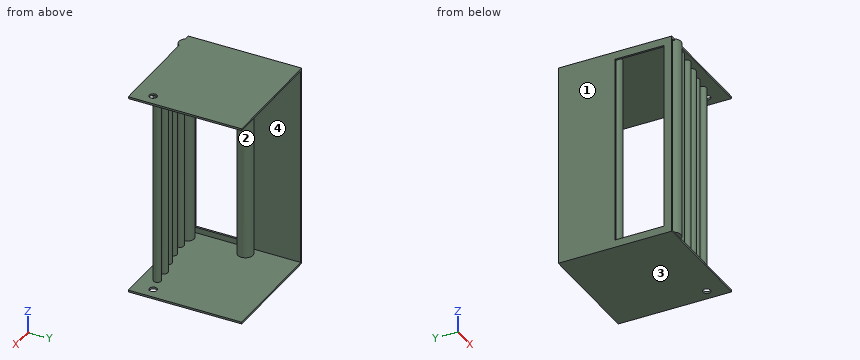
```python
from build123d import *

# Parameters (mm, degrees)
SKETCH1_W               = 381
SKETCH1_H               = 685.8
BOSS_EXTRUDE1_DEPTH     = 381
SHELL1_T                = -6.35
SKETCH4_R               = 12.7
CUT_EXTRUDE1_DEPTH      = 1
CUT_EXTRUDE1_DEPTH_BACK = 686.8
SKETCH5_R               = 12.7
BOSS_EXTRUDE3_DEPTH     = 679.45
SKETCH6_R               = 25.4
BOSS_EXTRUDE4_DEPTH     = 679.45
CUT_EXTRUDE3_REACH      = 8.35
SKETCH7_W               = 635
SKETCH7_H               = 165.1


with BuildPart() as part:
    # Sketch1 → Boss-Extrude1 (new body)
    with BuildSketch(Plane(origin=(0, 0, 0), x_dir=(1, 0, 0), z_dir=(0, 1, 0))):
        with Locations((190.5, 342.9)):
            Rectangle(SKETCH1_W, SKETCH1_H)
    extrude(amount=BOSS_EXTRUDE1_DEPTH)

    # Shell1
    shell1_openings = [part.faces().sort_by_distance(p)[0] for p in [
        (190.5, 381, -342.9),
        (190.5, 0, -342.9),
        (381, 190.5, -342.9),
    ]]
    offset(amount=SHELL1_T, openings=shell1_openings, kind=Kind.INTERSECTION)

    # Sketch4 → Cut-Extrude1 (cut, two sides)
    with BuildSketch(Plane.XY) as cut_extrude1_sk:
        with Locations((342.9, 63.5)):
            Circle(SKETCH4_R)
    extrude(amount=CUT_EXTRUDE1_DEPTH, mode=Mode.SUBTRACT)
    extrude(cut_extrude1_sk.sketch, amount=-CUT_EXTRUDE1_DEPTH_BACK, mode=Mode.SUBTRACT)

    # Sketch5 → Boss-Extrude3 (add)
    with BuildSketch(Plane.XY):
        with Locations((292.1, 50.8)):
            Circle(SKETCH5_R)
        with Locations((190.5, 32.743756917)):
            Circle(SKETCH5_R)
        with Locations((88.9, 19.34192219)):
            Circle(SKETCH5_R)
        with Locations((241.3, 46.355575893)):
            Circle(SKETCH5_R)
        with Locations((139.7, 23.786346297)):
            Circle(SKETCH5_R)
    extrude(amount=-BOSS_EXTRUDE3_DEPTH)

    # Sketch6 → Boss-Extrude4 (add)
    with BuildSketch(Plane.XY):
        with Locations((38.1, 14.897498083)):
            Circle(SKETCH6_R)
        with Locations((38.1, 211.747498083)):
            Circle(SKETCH6_R)
    extrude(amount=-BOSS_EXTRUDE4_DEPTH)

    # Sketch7 → Cut-Extrude3 (cut, up to next)
    with BuildSketch(Plane(origin=(6.35, 0, 0), x_dir=(0, 0, -1), z_dir=(1, 0, 0)), mode=Mode.PRIVATE) as cut_extrude3_sk1:
        with Locations((342.9, 107.95)):
            Rectangle(SKETCH7_W, SKETCH7_H)
    cut_extrude3_tool1 = extrude(cut_extrude3_sk1.sketch, amount=-CUT_EXTRUDE3_REACH, mode=Mode.PRIVATE) & part.part
    add(cut_extrude3_tool1.solids().sort_by_distance((6.35, 107.95, -342.9))[0], mode=Mode.SUBTRACT)


solid = part.part
```
Source: CAD feature listing. Evaluate the final solid. Frame: model axes, mm. Face numbers are marked on the shaded views. A direction names the side the tool comes from. Give positions to 0.01 mm unless a question says otherwise; leave off trailing zeros. Write each loop counter-clockwise with the first axis right and the second up, starting at its lowest first coordinate (ties: lowest second). Pieces come first, ordered by that corner, then holes.
1. Section query C-C (x = 38.1). Return the cut outline in (y, z), then the cut area to 3 significant figures.
2. Section query A-A (x = 169.5). Return the cut outline in (y, z), then the cut area to 3 significant figures.
3. Pull-direction query (Y, two-part tool) for the marked faces 1 and 2; classes: +Y half, -Y half, draft (parallel to the pull), parting line (faces both ways), or undercut.
4. Access query for the marked faces 3 and 4. Directions: +Z, -Z, +X, -X, +Y, -Y. A direction counts if a zero-diameter tool reaches every point of the face in a straight line with its end or side. Return the directions, or none.
5. Section query D-D (z = -623.5). Count the separate pieces of the cut face and the enclosed holes in it, then the cut area to 3 significant figures.
6. Material intervals for line 1 along Z through (x, y) = (63.5, 332); line 2 along X through (y, z) = (63, -681); line 3 along Y through (x, z) = (342.9, -680.75), sorted ascending.
7. First-contact query: pin 1 (4 mm diameter, centred on x = 61.5, z = -500.5, fed in from +Y); pin 2 (1.5 mm diameter, centred on x = 299, z = -573.5, fed in from +Y); pin 3 (5.5 mm diameter, centred on x = 42.5, y = -6.5, fed in from -Z). Flat tips, straight axial feed; report the tip coordinate or a pass-through.
8. Section query B-B (x = 342.9). Return the cut outline in (y, z).
Output values:
1. outline: (-10.5, -679.45) - (0, -679.45) - (0, -685.8) - (381, -685.8) - (381, -679.45) - (237.15, -679.45) - (237.15, -6.35) - (381, -6.35) - (381, 0) - (-10.5, 0) - close; hole (40.3, -679.45) - (186.35, -679.45) - (186.35, -6.35) - (40.3, -6.35) - close
1. area: 73,300 mm2
2. outline: (0, -685.8) - (381, -685.8) - (381, -679.45) - (0, -679.45) - close; (0, -6.35) - (381, -6.35) - (381, 0) - (0, 0) - close
2. area: 4,840 mm2
3. face 1: draft
3. face 2: undercut
4. face 3: -Z, +X, -X, +Y, -Y
4. face 4: +Y, -Y
5. separate pieces: 9
5. enclosed holes: 0
5. area: 7,960 mm2
6. line 1: z = -685.8 to -679.45, -6.35 to 0
6. line 2: x = 0 to 330.21, 355.59 to 381
6. line 3: y = 0 to 50.8, 76.2 to 381
7. pin 1: stops at y = 225.43
7. pin 2: stops at y = 61.91
7. pin 3: stops at z = -679.45
8. outline: (0, -685.8) - (50.8, -685.8) - (50.8, -679.45) - (0, -679.45) - close; (0, -6.35) - (50.8, -6.35) - (50.8, 0) - (0, 0) - close; (76.2, -685.8) - (381, -685.8) - (381, -679.45) - (76.2, -679.45) - close; (76.2, -6.35) - (381, -6.35) - (381, 0) - (76.2, 0) - close
